Here's how the part is built. I have some questions about the finished solid (model axes, mm). A direction names the side the tool comes from. Coordinates: 2 decimals unless noted, no trailing zeros. Write each loop counter-clockwise with the first axis right and the second up, starting at its lowest first coordinate (ties: lowest second). Pieces come first, ordered by that corner, then holes. Notation, with made-up numbers: (77.25, 3) -> (127.25, 3) arc R31 ccw to (127.25, 36) -> close; hole circle Ø1 at (46.5, 28). An arc over 180 degrees is marked (long way). Put each result on its own line as item: value.
```python
from build123d import *

# Parameters (mm, degrees)
SKETCH_R     = 1.5
PAD_DEPTH    = 1.5
SKETCH001_W  = 26.8
SKETCH001_H  = 19.2
PAD001_DEPTH = 1.75


with BuildPart() as part:
    # Sketch → Pad (new body, symmetric)
    with BuildSketch(Plane.XY):
        with BuildLine():
            Line((-14.05, 17.85), (14.05, 17.85))
            ThreePointArc((17.85, 14.05), (16.737006, 16.737006), (14.05, 17.85))
            Line((17.85, 14.05), (17.85, -14.05))
            ThreePointArc((14.05, -17.85), (16.737006, -16.737006), (17.85, -14.05))
            Line((14.05, -17.85), (-14.05, -17.85))
            ThreePointArc((-17.85, -14.05), (-16.737006, -16.737006), (-14.05, -17.85))
            Line((-17.85, -14.05), (-17.85, 14.05))
            ThreePointArc((-14.05, 17.85), (-16.737006, 16.737006), (-17.85, 14.05))
        make_face()
        with Locations((-14, 14)):
            Circle(SKETCH_R, mode=Mode.SUBTRACT)
        with Locations((-14, -14)):
            Circle(SKETCH_R, mode=Mode.SUBTRACT)
        with Locations((14, -14)):
            Circle(SKETCH_R, mode=Mode.SUBTRACT)
        with Locations((14, 14)):
            Circle(SKETCH_R, mode=Mode.SUBTRACT)
    extrude(amount=PAD_DEPTH, both=True)

    # Sketch001 → Pad001 (new body)
    with BuildSketch(Plane.XY.offset(1.5)):
        with Locations((0.15, -0.3)):
            Rectangle(SKETCH001_W, SKETCH001_H)
    extrude(amount=PAD001_DEPTH)


solid = part.part
```
Item 1: Imagine slicing it at D-D on y = 3. Write out the boundary of the cut face in (x, z).
Output:
outline: (-17.85, -1.5) -> (17.85, -1.5) -> (17.85, 1.5) -> (13.55, 1.5) -> (13.55, 3.25) -> (-13.25, 3.25) -> (-13.25, 1.5) -> (-17.85, 1.5) -> close
Item 2: Please list where these lines run through material, in increasing order: line 1 along Y through (x, z) = (-14, -0.9); line 2 along Y through (x, z) = (15, 0.9); line 3 along Z through (x, y) = (-14, -5). Write a range as from..to.
Output:
line 1: y = -17.85..-15.5, -12.5..12.5, 15.5..17.85
line 2: y = -17.73..-15.12, -12.88..12.88, 15.12..17.73
line 3: z = -1.5..1.5
Item 3: If we mould it in two halves opening along X, with no side actions, what happens to faces 5 (the flat face through (-13.25, 0, 2)), 6 (the flat face through (0, -17.85, 0)), 7 (the cylindrical face through (16.766, 16.707, 0.021)), 8 (the cylindrical face through (-15.5, 14.07, -0.02))? For each: released by +X, released by -X, zero draft, split by the parting line, or undercut.
Output:
face 5: released by -X
face 6: zero draft
face 7: released by +X
face 8: undercut
Item 4: Imagine slicing it at B-B on y = 13. Write out the boundary of the cut face in (x, z), then the cut area to 3 significant figures.
Output:
outline: (-17.85, -1.5) -> (-15.12, -1.5) -> (-15.12, 1.5) -> (-17.85, 1.5) -> close; (-12.88, -1.5) -> (12.88, -1.5) -> (12.88, 1.5) -> (-12.88, 1.5) -> close; (15.12, -1.5) -> (17.85, -1.5) -> (17.85, 1.5) -> (15.12, 1.5) -> close
area: 93.7 mm²
Item 5: Which directions (+Z, -Z, +X, -X, +Y, -Y) give clear straight access to the entire face, cutting with the end or side of a thin tool? Please do faces 1 (the flat face through (0, 9.3, 2)), 2 (the flat face through (0, -9.9, 2)), 3 (the flat face through (17.85, 0, 0)), 4 (the flat face through (13.55, 0, 2)).
Output:
face 1: +Z, +X, -X, +Y
face 2: +Z, +X, -X, -Y
face 3: +Z, -Z, +X, +Y, -Y
face 4: +Z, +X, +Y, -Y
Item 6: For P1, Ø0.9, axis at x = -1, z = 2.5, coming from the -Y side; P2, Ø4, axis at x = -14, y = 14, coming from the +Z side; P3, Ø1.4, axis at x = 0.5, z = 2, coming from the +Y side; P4, Ø2.5, axis at x = -14, y = -14, coming from the +Z side, each with a flat end and sliding along its axis, tell me the tip position at first contact or that it passes through.
Output:
P1: stops at y = -9.9
P2: stops at z = 1.5
P3: stops at y = 17.85
P4: passes through
Item 7: Imagine slicing it at C-C on x = 10. Write out the boundary of the cut face in (y, z), then the cut area to 3 significant figures.
Output:
outline: (-17.85, -1.5) -> (17.85, -1.5) -> (17.85, 1.5) -> (9.3, 1.5) -> (9.3, 3.25) -> (-9.9, 3.25) -> (-9.9, 1.5) -> (-17.85, 1.5) -> close
area: 141 mm²
Item 8: Imagine slicing it at A-A on z = 0.9. Write out the boundary of the cut face in (x, y), then the cut area to 3 significant figures.
Output:
outline: (-17.85, -14.05) arc R3.8 ccw to (-14.05, -17.85) -> (14.05, -17.85) arc R3.8 ccw to (17.85, -14.05) -> (17.85, 14.05) arc R3.8 ccw to (14.05, 17.85) -> (-14.05, 17.85) arc R3.8 ccw to (-17.85, 14.05) -> close; hole circle Ø3 at (-14, -14); hole circle Ø3 at (-14, 14); hole circle Ø3 at (14, -14); hole circle Ø3 at (14, 14)
area: 1,230 mm²
